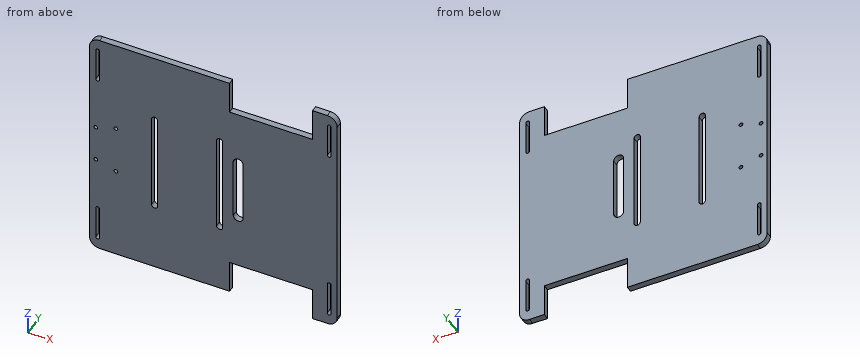
from build123d import *

# Parameters (mm, degrees)
SKETCH2_W           = 200
SKETCH2_H           = 195
BOSS_EXTRUDE1_DEPTH = 5
CUT_EXTRUDE1_DEPTH  = 140.754248594
SKETCH4_W           = 67
SKETCH4_H           = 27
CUT_EXTRUDE2_DEPTH  = 140.754248594
SKETCH8_R           = 1.5
CUT_EXTRUDE6_DEPTH  = 140.754248594
SKETCH9_R           = 1.5
CUT_EXTRUDE7_DEPTH  = 140.754248594
FILLET1_R           = 8


with BuildPart() as part:
    # Sketch2 → Boss-Extrude1 (new body)
    with BuildSketch(Plane(origin=(0, 0, 0), x_dir=(1, 0, 0), z_dir=(0, 1, 0))):
        Rectangle(SKETCH2_W, SKETCH2_H)
    extrude(amount=BOSS_EXTRUDE1_DEPTH)

    # Sketch3 → Cut-Extrude1 (cut, through all)
    with BuildSketch(Plane(origin=(0, 5, 0), x_dir=(1, 0, 0), z_dir=(0, 1, 0))):
        with BuildLine():
            Line((-95, -87.5), (-95, -60.5))
            ThreePointArc((-95, -60.5), (-93.5, -59), (-92, -60.5))
            Line((-92, -60.5), (-92, -87.5))
            ThreePointArc((-92, -87.5), (-93.5, -89), (-95, -87.5))
        make_face()
        with BuildLine():
            Line((-95, 87.5), (-95, 60.5))
            ThreePointArc((-95, 60.5), (-93.5, 59), (-92, 60.5))
            Line((-92, 60.5), (-92, 87.5))
            ThreePointArc((-92, 87.5), (-93.5, 89), (-95, 87.5))
        make_face()
        with BuildLine():
            Line((95, 87.5), (95, 60.5))
            ThreePointArc((95, 60.5), (93.5, 59), (92, 60.5))
            Line((92, 60.5), (92, 87.5))
            ThreePointArc((92, 87.5), (93.5, 89), (95, 87.5))
        make_face()
        with BuildLine():
            Line((95, -87.5), (95, -60.5))
            ThreePointArc((95, -60.5), (93.5, -59), (92, -60.5))
            Line((92, -60.5), (92, -87.5))
            ThreePointArc((92, -87.5), (93.5, -89), (95, -87.5))
        make_face()
    extrude(amount=-CUT_EXTRUDE1_DEPTH, mode=Mode.SUBTRACT)

    # Sketch4 → Cut-Extrude2 (cut, through all)
    with BuildSketch(Plane.XZ):
        with Locations((46.5, -84)):
            Rectangle(SKETCH4_W, SKETCH4_H)
        with Locations((46.5, 84)):
            Rectangle(SKETCH4_W, SKETCH4_H)
        with BuildLine():
            Line((-45, 40), (-45, -40))
            ThreePointArc((-45, -40), (-47.5, -42.5), (-50, -40))
            Line((-50, -40), (-50, 40))
            ThreePointArc((-50, 40), (-47.5, 42.5), (-45, 40))
        make_face()
        with BuildLine():
            Line((24, 25), (24, -25))
            ThreePointArc((24, -25), (20, -29), (16, -25))
            Line((16, -25), (16, 25))
            ThreePointArc((16, 25), (20, 29), (24, 25))
        make_face()
        with BuildLine():
            Line((7.5, 40), (7.5, -40))
            ThreePointArc((7.5, -40), (5, -42.5), (2.5, -40))
            Line((2.5, -40), (2.5, 40))
            ThreePointArc((2.5, 40), (5, 42.5), (7.5, 40))
        make_face()
    extrude(amount=-CUT_EXTRUDE2_DEPTH, mode=Mode.SUBTRACT)

    # Sketch8 → Cut-Extrude6 (cut, through all)
    with BuildSketch(Plane(origin=(0, 5, 0), x_dir=(1, 0, 0), z_dir=(0, 1, 0))):
        with Locations(Location((-78.75, 19.995, 0), (0, 0, 270))):
            Circle(SKETCH8_R)
        with Locations(Location((-78.75, -19.995, 0), (0, 0, 270))):
            Circle(SKETCH8_R)
    extrude(amount=-CUT_EXTRUDE6_DEPTH, mode=Mode.SUBTRACT)

    # Sketch9 → Cut-Extrude7 (cut, through all)
    with BuildSketch(Plane(origin=(0, 5, 0), x_dir=(1, 0, 0), z_dir=(0, 1, 0))):
        with Locations(Location((-95, 15, 0), (0, 0, 270))):
            Circle(SKETCH9_R)
        with Locations(Location((-95, -15, 0), (0, 0, 90))):
            Circle(SKETCH9_R)
    extrude(amount=-CUT_EXTRUDE7_DEPTH, mode=Mode.SUBTRACT)

    # Fillet1
    fillet1_edges = [part.edges().sort_by_distance(p)[0] for p in [
        (100, 2.5, 97.5),
        (-100, 2.5, 97.5),
        (-100, 2.5, -97.5),
        (100, 2.5, -97.5),
    ]]
    fillet(fillet1_edges, radius=FILLET1_R)


solid = part.part
Input: part model. Units: mm. Frame: model coordinates. Round coordinates to 2 decimals unless told otherwise and drop trailing zeros. Loops run counter-clockwise (first coordinate to the right, second up) from the corner with the lowest first, then second, coordinate; pieces in that order, holes last. Notation, with made-up numbers: M 85,26.5 L 124,26.5 A16 cw 124,55.5 Z; hole C 67,-9 d2. An arc over 180 degrees is marked long. Answer as CSV lines item,"result". Start each with the question number.
(1) Section D-D, the plane y = 1.6. State how many separate pieces and enclosed holes the cut face has, plus the area to 3 significant figures.
(2) First-contact query: pin 1 (1.5 mm diameter, centred on x = 17.5, y = 4, fed in from +Z). Flat tip, straight axial feed; report the tip coordinate or a pass-through.
(3) Line query: line 1 (Z direction, x = -78.75, y = 2.85) (3 decimals); line 2 (X direction, y = 1, z = -5.5); line 3 (X direction, y = 1.1, z = 61.5). Output: solid intervals per line, ascending. Write a range as [from, to].
(4) Section A-A, the plane z = -3.5. Output: boundary loops of the cut face in (x, y).
(5) Section C-C, the plane x = 20.5. Output: boundary loops of the cut face in (y, z).
(6) Section B-B, the plane z = -66. Output: boundary loops of the cut face in (x, y).
Values found:
1,separate pieces,"1"
1,enclosed holes,"11"
1,area,"33,700 mm²"
2,pin 1,"stops at z = 70.5"
3,line 1,"z = [-97.5, -21.495], [-18.495, 18.495], [21.495, 97.5]"
3,line 2,"x = [-100, -50], [-45, 2.5], [7.5, 16], [24, 100]"
3,line 3,"x = [-100, -95], [-92, 92], [95, 100]"
4,outline,"M -100,0 L -50,0 L -50,5 L -100,5 Z; M -45,0 L 2.5,0 L 2.5,5 L -45,5 Z; M 7.5,0 L 16,0 L 16,5 L 7.5,5 Z; M 24,0 L 100,0 L 100,5 L 24,5 Z"
5,outline,"M 0,-70.5 L 5,-70.5 L 5,-28.97 L 0,-28.97 Z; M 0,28.97 L 5,28.97 L 5,70.5 L 0,70.5 Z"
6,outline,"M -100,0 L -95,0 L -95,5 L -100,5 Z; M -92,0 L 92,0 L 92,5 L -92,5 Z; M 95,0 L 100,0 L 100,5 L 95,5 Z"
